Check sheet for the modelled part. Datum: model origin and axes. Units: mm. Face numbers are marked on the shaded views. A direction names the side the tool comes from. Coordinates: 2 decimals unless noted, no trailing zeros. Write each loop counter-clockwise with the first axis right and the second up, starting at its lowest first coordinate (ties: lowest second). Pieces come first, ordered by that corner, then holes. Notation, with made-up numbers: (68.5, 65) -> (116.5, 65) arc R7 ccw to (116.5, 71) -> close; hole circle Ø10 at (-3.5, 0.5). An arc over 180 degrees is marked (long way). Put each result on its own line as item: value.
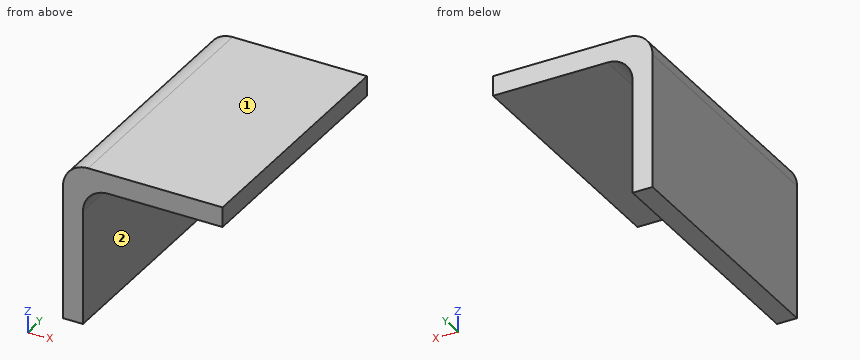
```python
from build123d import *

# Parameters (mm, degrees)
BOSS_EXTRUDE1_DEPTH = 20.32
FILLET1_R           = 2
FILLET2_R           = 2


with BuildPart() as part:
    # Sketch1 → Boss-Extrude1 (new body)
    with BuildSketch(Plane(origin=(0, 0, 0), x_dir=(1, 0, 0), z_dir=(0, 1, 0))):
        Polygon((-7.943330105, 9.7977882), (-6.353330105, 9.7977882), (-6.353330105, -1.3147118), (4.756669895, -1.3147118), (4.756669895, -2.9022118), (-6.353330105, -2.9022118), (-7.943330105, -2.9022118), align=None)
    extrude(amount=BOSS_EXTRUDE1_DEPTH)

    # Fillet1
    fillet1_edges = [part.edges().sort_by_distance(p)[0] for p in [
        (-6.353330105, 10.16, 1.3147118),
    ]]
    fillet(fillet1_edges, radius=FILLET1_R)

    # Fillet2
    fillet2_edges = [part.edges().sort_by_distance(p)[0] for p in [
        (-7.943330105, 10.16, 2.9022118),
    ]]
    fillet(fillet2_edges, radius=FILLET2_R)


solid = part.part
```
Q1. Material ranges on line 1 along X through (y, z) = (10.75, -2.75); line 2 along Z through (x, y) = (-3.75, 17.25); line 3 along Z through (x, y) = (-5.75, 2.75), recorded low to high.
Recorded:
line 1: x = -7.94 to -6.35
line 2: z = 1.31 to 2.9
line 3: z = 0.75 to 2.9
Q2. Cross-section at B-B (z = -7). Record the cut outline in (x, y), plus the area to 3 significant figures.
Recorded:
outline: (-7.94, 0) -> (-6.35, 0) -> (-6.35, 20.32) -> (-7.94, 20.32) -> close
area: 32.3 mm2
Q3. Cross-section at C-C (x = -2.25). Record the cut outline in (y, z), plus the area to 3 significant figures.
Recorded:
outline: (0, 1.31) -> (20.32, 1.31) -> (20.32, 2.9) -> (0, 2.9) -> close
area: 32.3 mm2
Q4. Tool access check on the marked faces 1 and 2. Record the directions out of +Z, -Z, +X, -X, +Y, -Y that give a thin tool (end or side, any length) a straight path to the whole face; none if there is none.
Recorded:
face 1: +Z, +X, -X, +Y, -Y
face 2: -Z, +X, +Y, -Y
Q5. Cross-section at A-A (y = 11). Record the cut outline in (x, z).
Recorded:
outline: (-7.94, -9.8) -> (-6.35, -9.8) -> (-6.35, -0.69) arc R2 cw to (-4.35, 1.31) -> (4.76, 1.31) -> (4.76, 2.9) -> (-5.94, 2.9) arc R2 ccw to (-7.94, 0.9) -> close
Q6. Depth check by flat-ended pin: P1, Ø7.5, axis at y = 14, z = -4, coming from the +X side; P2, Ø3, axis at x = 0, y = 11, coming from the -Z side; P3, Ø4, axis at y = 16.5, z = -6, coming from the +X side. Enter the tip coordinate at first touch or a pass-through.
Recorded:
P1: stops at x = -6.31
P2: stops at z = 1.31
P3: stops at x = -6.35
